Check sheet for the modelled part. Datum: model origin and axes. Units: mm. Round coordinates to 2 decimals unless told otherwise and drop trailing zeros. Loops run counter-clockwise (first coordinate to the right, second up) from the corner with the lowest first, then second, coordinate; pieces in that order, holes last. Notation, with made-up numbers: (20.25, -15.75) -> (79.25, -15.75) arc R30 cw to (79.25, 16.25) -> close; hole circle Ø9 at (-35, 19.25). An arc over 180 degrees is marked (long way). One line per item, written item: value. Start each with the question number.
1. Go/stop test with flat-tipped pins: pin 1 (1.5 mm diameter, centred on x = 3.5, y = 1.5, fed in from +Z); pin 2 (1.5 mm diameter, centred on y = 0.5, z = -9.5, fed in from +X); pin 3 (1 mm diameter, centred on y = 1.5, z = -5, fed in from +X). Record where each tip stops, or that it passes through.
2. Cross-section at A-A on y = 0.95. Record the cut outline in (x, z).
3. Cross-section at C-C on x = 22.75. Record the cut outline in (y, z) (3 decimals).
4. Material ranges on L1, parallel to Z at x = 2.25, y = 1.65; L2, parallel to Z at x = 6.5, y = 1.35; L3, parallel to X at y = 1.75, z = -10.75, recorded low to high.
5. Cross-section at B-B on z = -6. Record the cut outline in (x, y) (3 decimals).
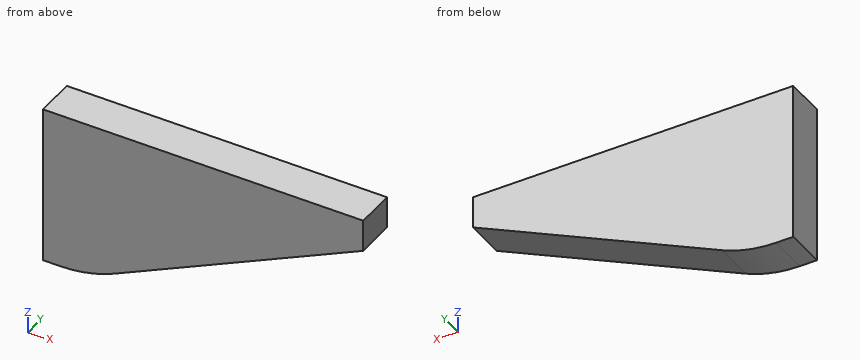
from build123d import *

# Parameters (mm, degrees)
SKETCH1_W           = 25.4
SKETCH1_H           = 12.7
BOSS_EXTRUDE1_DEPTH = 3.175
CHAMFER1_SIZE       = 10.16
CHAMFER1_SIZE2      = 21.788190312
FILLET1_R           = 10.16


with BuildPart() as part:
    # Sketch1 → Boss-Extrude1 (new body)
    with BuildSketch(Plane(origin=(0, 0, 0), x_dir=(1, 0, 0), z_dir=(0, 1, 0))):
        with Locations((12.7, 6.35)):
            Rectangle(SKETCH1_W, SKETCH1_H)
    extrude(amount=BOSS_EXTRUDE1_DEPTH)

    # Chamfer1
    chamfer1_edges = [part.edges().sort_by_distance(p)[0] for p in [
        (25.4, 1.5875, -12.7),
    ]]
    chamfer1_side = [part.faces().sort_by_distance(p)[0] for p in [
        (25.4, 1.5875, -6.35),
    ]]
    chamfer(chamfer1_edges, length=CHAMFER1_SIZE, length2=CHAMFER1_SIZE2, reference=chamfer1_side[0])

    # Fillet1
    fillet1_edges = [part.edges().sort_by_distance(p)[0] for p in [
        (3.611809688, 1.5875, -12.7),
    ]]
    fillet(fillet1_edges, radius=FILLET1_R)


solid = part.part
Taken from the geometry:
1. pin 1: stops at z = 0
1. pin 2: stops at x = 12.08
1. pin 3: stops at x = 21.2
2. outline: (0, -12.7) -> (1.36, -12.7) arc R10.16 ccw to (5.65, -11.75) -> (25.4, -2.54) -> (25.4, 0) -> (0, 0) -> close
3. outline: (0, -3.776) -> (3.175, -3.776) -> (3.175, 0) -> (0, 0) -> close
4. L1: z = -12.66 to 0
4. L2: z = -11.35 to 0
4. L3: x = 0 to 7.79
5. outline: (0, 0) -> (17.98, 0) -> (17.98, 3.175) -> (0, 3.175) -> close
